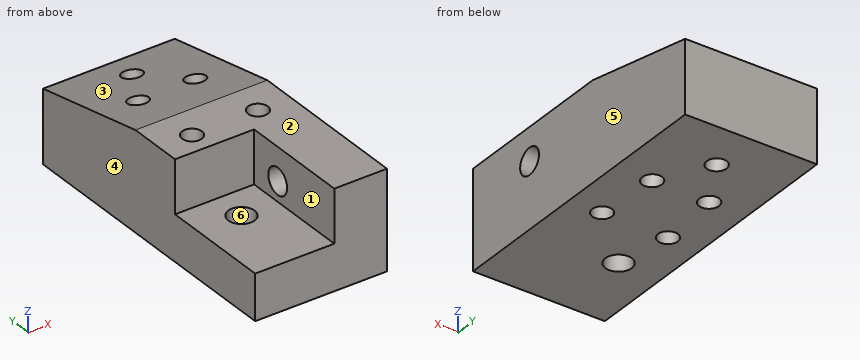
Autodesk Inventor part; units mm, degrees
ref_plane "YZ Plane" through (0, 0, 0) normal (1, 0, 0) x (0, 1, 0)
ref_plane "XZ Plane" through (0, 0, 0) normal (0, 1, 0) x (-1, 0, 0)
ref_plane "XY Plane" through (0, 0, 0) normal (0, 0, 1) x (1, 0, 0)
sketch "Sketch1" plane through (0, 0, 0) normal (1, 0, 0) x (0, 1, 0)
  line L0 (0, 0) -> (19.6116, -3.9223)
  line L1 (0, 0) -> (20, 0) construction
  line L2 (19.6116, -3.9223) -> (19.6116, -14.9223)
  line L3 (19.6116, -14.9223) -> (-10.3884, -14.9223)
  line L4 (-10.3884, -14.9223) -> (-10.3884, 0)
  line L5 (-10.3884, 0) -> (0, 0)
  dimension "d0" = 20
  dimension "d1" = 11.31
  dimension "d2" = 11
  dimension "d3" = 30
extrude "Extrusion1" add sketch "Sketch1" along normal blind 20
sketch "Sketch2" plane through (0, 0, 0) normal (0, 0.1961, 0.9806) x (1, 0, 0)
  line L0 (0, 0) -> (10, 0)
  line L1 (0, 0) -> (20, 0)
  line L2 (10, 0) -> (10, 15)
  circle A0 centre (10, 15) radius 1.5
  line L3 (10, 15) -> (10, 10)
  circle A1 centre (5.6699, 7.5) radius 1.5
  circle A2 centre (14.3301, 7.5) radius 1.5
  dimension "d6" = 15
  dimension "d7" = 3
  dimension "d8" = 5
  dimension "d11" = 360
extrude "Extrusion2" cut sketch "Sketch2" against normal blind 20
sketch "Sketch3" plane through (0, -10.3884, 0) normal (0, 0, 1) x (1, 0, 0)
  line L0 (0, 10.3884) -> (0, 0)
  line L1 (0, 10.3884) -> (0, 5.3884)
  line L2 (0, 5.3884) -> (5, 5.3884)
  line L3 (5, 5.3884) -> (15, 5.3884)
  circle A0 centre (5, 5.3884) radius 1.5
  circle A1 centre (15, 5.3884) radius 1.5
  dimension "d15" = 5
  dimension "d16" = 5
  dimension "d17" = 10
  dimension "d18" = 3
  dimension "d19" = 3
extrude "Extrusion3" cut sketch "Sketch3" against normal blind 20
sketch "Sketch4" plane through (20, 0, 0) normal (1, 0, 0) x (0, 0, -1)
  line L0 (14.9223, -10.3884) -> (14.9223, 19.6116)
  line L1 (0, -10.3884) -> (14.9223, -10.3884)
  line L2 (14.9223, -10.3884) -> (0, -10.3884)
  point P0 (0, 0)
sketch "Sketch5" plane through (20, 0, 0) normal (1, 0, 0) x (0, 0, -1)
  line L0 (0, 0) -> (0, -10.3884)
  line L1 (0, -10.3884) -> (14.9223, -10.3884)
  line L2 (14.9223, -10.3884) -> (14.9223, -25.3884)
  line L3 (14.9223, -25.3884) -> (0, -25.3884)
  line L4 (0, -25.3884) -> (0, -10.3884)
  dimension "d22" = 15
  dimension "d25" = 14.9223
extrude "Extrusion4" add sketch "Sketch5" against normal blind 20
sketch "Sketch10" plane through (0, 0, 0) normal (0, 0, 1) x (1, 0, 0)
  line L0 (0, -25.3884) -> (0, 19.6116)
  line L1 (0, -25.3884) -> (12, -25.3884)
  line L2 (12, -25.3884) -> (12, -8.3884)
  line L3 (12, -8.3884) -> (0, -8.3884)
  line L4 (0, -8.3884) -> (0, -25.3884)
  point P0 (0, 0)
  point P1 (0, -8.3884)
  dimension "d39" = 12
  dimension "d40" = 17
extrude "Extrusion8" cut sketch "Sketch10" against normal blind 8
sketch "Sketch11" plane through (20, 0, 0) normal (1, 0, 0) x (0, 0, -1)
  line L0 (0, -25.3884) -> (8, -25.3884)
  line L1 (0, -25.3884) -> (5, -25.3884)
  line L2 (5, -25.3884) -> (5, -13.3884)
  circle A0 centre (5, -13.3884) radius 2
  point P0 (0, 0)
  dimension "d43" = 5
  dimension "d44" = 12
  dimension "d45" = 4
extrude "Extrusion9" cut sketch "Sketch11" against normal blind 8
sketch "Sketch12" plane through (20, 19.6116, -14.9223) normal (0, 0, -1) x (-1, 0, 0)
  line L0 (20, -45) -> (20, 0)
  line L1 (20, -45) -> (13.5, -45)
  line L2 (8, -45) -> (20, -45)
  line L3 (13.5, -45) -> (13.5, -33)
  circle A0 centre (13.5, -33) radius 2
  point P0 (20, -19.6116)
  dimension "d48" = 6.5
  dimension "d49" = 12
  dimension "d50" = 4
extrude "Extrusion10" cut sketch "Sketch12" against normal blind 8
properties part number "connector"
For this review, take the finished solid that the model builds, in its own axes (mm). Face numbers are marked on the shaded views. A direction names the side the tool comes from. Coordinates: 2 decimals unless noted, no trailing zeros. Order: outer loops, then holes, each group sorted by start corner. A loop starts at its lowest first (then second) coordinate and runs counter-clockwise, first axis right, second up. Notation, with made-up numbers: (54, 54) -> (74, 54) arc R9 ccw to (74, 71) -> close; hole circle Ø6 at (-15, 12.5). An arc over 180 degrees is marked (long way). Answer as CSV lines item,"result".
Q1. Clearance check with flat-ended pins moving along their axes: pin 1 Ø4.5 at (y, z) = (-13.39, -5) entering from -X; pin 2 Ø1.5 at (x, y) = (15.5, 12.5) entering from +Z; pin 3 Ø3.5 at (x, y) = (8, -15.5) entering from +Z. State where each tip first meets the part, or that it passes through.
Model answer:
pin 1,"stops at x = 12"
pin 2,"stops at z = -2.35"
pin 3,"stops at z = -8"
Q2. We need section B-B (x = 15). State the section outline as (y, z) points.
Model answer:
outline,"(-25.39, -14.92) -> (-6.5, -14.92) -> (-6.5, 0) -> (-25.39, 0) -> close; (-3.5, -14.92) -> (3.3, -14.92) -> (6.04, -1.21) -> (0, 0) -> (-3.5, 0) -> close; (6.03, -14.92) -> (19.61, -14.92) -> (19.61, -3.92) -> (8.67, -1.73) -> close; hole circle Ø4 at (-13.39, -5)"
Q3. We need section C-C (x = 2.75). State the section outline as (y, z) points.
Model answer:
outline,"(-25.39, -14.92) -> (19.61, -14.92) -> (19.61, -3.92) -> (0, 0) -> (-8.39, 0) -> (-8.39, -8) -> (-25.39, -8) -> close"
Q4. Wall thickness on line 1 along X through (y, z) = (-5, -4.75); line 2 along Y through (x, z) = (5, -5.75); line 3 along Y through (x, z) = (15, -6.75): over which ranges is each line inside the solid? List them lowest first. Write a range as [from, to].
Model answer:
line 1,"x = [0, 3.5], [6.5, 13.5], [16.5, 20]"
line 2,"y = [-8.39, -6.5], [-3.5, 5.13], [7.87, 19.61]"
line 3,"y = [-25.39, -14.36], [-12.42, -6.5], [-3.5, 4.93], [7.67, 19.61]"
Q5. We need section A-A (y = -5). State the section outline as (x, z) points.
Model answer:
outline,"(0, -14.92) -> (3.5, -14.92) -> (3.5, 0) -> (0, 0) -> close; (6.5, -14.92) -> (13.5, -14.92) -> (13.5, 0) -> (6.5, 0) -> close; (16.5, -14.92) -> (20, -14.92) -> (20, 0) -> (16.5, 0) -> close"
Q6. Draft analysis for pull direction X (two halves, no side actions). For the marked faces 3, 4, 5 and 6, state which applies: released by +X, released by -X, zero draft, split by the parting line, or undercut.
Model answer:
face 3,"zero draft"
face 4,"released by -X"
face 5,"released by +X"
face 6,"undercut"
Q7. For the marked faces 1 and 2, list the 3-axis set-ups (+Z, -Z, +X, -X, +Y, -Y) from which the entire face can be reached by the end or side of a thin tool; tool diameter is ignored.
Model answer:
face 1,"+Z, -X, -Y"
face 2,"+Z, +X, -X, +Y, -Y"
